Geometry: final body of the model. Coordinates: model frame, mm. Face numbers are marked on the shaded views. Coordinates: 2 decimals unless noted, no trailing zeros. Write each loop counter-clockwise with the first axis right and the second up, starting at its lowest first coordinate (ties: lowest second). Pieces come first, ordered by that corner, then holes. Notation, with made-up numbers: (57.25, -17) - (96.25, -17) arc R22 ccw to (96.25, 17) - close; hole circle Ø10 at (-7, 30.25). An arc over 180 degrees is marked (long way). Answer as a JSON object with one key per item and string values. Group by question number.
Item 1: First-contact query: pin 1 Ø4 at (x, y) = (-17, -8.5) entering from -Z; pin 2 Ø0.9 at (y, z) = (5.5, 3) entering from -X; pin 3 Ø1.5 at (x, z) = (-47, 3) entering from -Y; pin 4 Ø0.9 at (y, z) = (-6, 3.5) entering from +X. Flat tips, straight axial feed; report the tip coordinate or a pass-through.
Item 2: Section D-D on y = 37. Return loops of the section in (x, z), and give its area (3 significant figures).
Item 3: Section A-A on x = 0. Return loops of the section in (y, z).
Item 4: Line query: line 1 along X through (y, z) = (-54.5, 3.25); line 2 along X through (y, z) = (-43, 0.65); line 3 along Y through (x, z) = (40, 0.7). Output: solid intervals per line, ascending. Write a range as from..to.
Item 5: Section C-C on y = -42. Return loops of the section in (x, z).
Item 6: Section B-B on z = 4.05. State how many separate pieces and enclosed holes the cut face has, and give its area (3 significant figures).
Item 7: Mould query, pull axis Z, two halves, no side actions, for the marked faces 1 and 2. Classes: pulls with the +Z half, pulls with the -Z half, needs draft (parallel to the pull), parting line crosses it, or undercut.
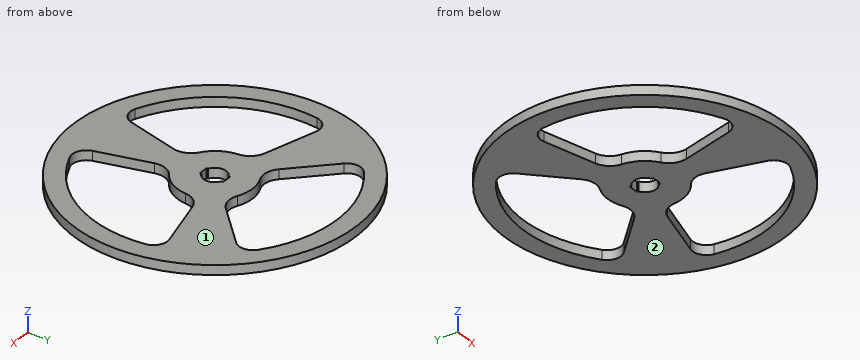
```python
from build123d import *

# Parameters (mm, degrees)
SKETCH1_R          = 75
SKETCH1_R_2        = 6
EXTRUSION1_DEPTH   = 5.1
CUT_EXTRUDE1_DEPTH = 107.188558706


with BuildPart() as part:
    # Sketch1 → Extrusion1 (new body)
    with BuildSketch(Plane.XY):
        Circle(SKETCH1_R)
        Circle(SKETCH1_R_2, mode=Mode.SUBTRACT)
        with BuildLine():
            ThreePointArc((40.502817464, 40.06150101), (42.745132776, 45.851099569), (39.856206804, 51.346691998))
            ThreePointArc((39.856206804, 51.346691998), (0, 65), (-39.856206804, 51.346691998))
            ThreePointArc((-39.856206804, 51.346691998), (-42.506769406, 45.932667816), (-40.316594862, 40.316594862))
            Line((-40.316594862, 40.316594862), (-20, 20))
            ThreePointArc((-20, 20), (-14.619951975, 17.215082215), (-8.619288125, 18.047378541))
            ThreePointArc((-8.619288125, 18.047378541), (0, 20), (8.619288125, 18.047378541))
            ThreePointArc((8.619288125, 18.047378541), (14.566416982, 17.206046598), (19.922803859, 19.923637571))
            Line((19.922803859, 19.923637571), (40.502817464, 40.06150101))
        make_face(mode=Mode.SUBTRACT)
        with BuildLine():
            ThreePointArc((-54.945686321, 15.045718344), (-61.080783406, 14.092821088), (-64.395643073, 8.843141592))
            ThreePointArc((-64.395643073, 8.843141592), (-56.291651246, -32.5), (-24.539436269, -60.18983359))
            ThreePointArc((-24.539436269, -60.18983359), (-18.525472489, -59.778276047), (-14.756897914, -55.073492776))
            Line((-14.756897914, -55.073492776), (-7.320508076, -27.320508076))
            ThreePointArc((-7.320508076, -27.320508076), (-7.598722539, -21.26879092), (-11.319844226, -16.48821175))
            ThreePointArc((-11.319844226, -16.48821175), (-17.320508076, -10), (-19.939132351, -1.559166791))
            ThreePointArc((-19.939132351, -1.559166791), (-22.184081943, 4.011863849), (-27.215778201, 7.291835471))
            Line((-27.215778201, 7.291835471), (-54.945686321, 15.045718344))
        make_face(mode=Mode.SUBTRACT)
        with BuildLine():
            ThreePointArc((14.442868856, -55.107219354), (18.33565063, -59.943920657), (24.539436269, -60.18983359))
            ThreePointArc((24.539436269, -60.18983359), (56.291651246, -32.5), (64.395643073, 8.843141592))
            ThreePointArc((64.395643073, 8.843141592), (61.032241895, 13.845608231), (55.073492776, 14.756897914))
            Line((55.073492776, 14.756897914), (27.320508076, 7.320508076))
            ThreePointArc((27.320508076, 7.320508076), (22.218674514, 4.053708705), (19.939132351, -1.559166791))
            ThreePointArc((19.939132351, -1.559166791), (17.320508076, -10), (11.319844226, -16.48821175))
            ThreePointArc((11.319844226, -16.48821175), (7.617664962, -21.217910447), (7.292974343, -27.215473042))
            Line((7.292974343, -27.215473042), (14.442868856, -55.107219354))
        make_face(mode=Mode.SUBTRACT)
    extrude(amount=EXTRUSION1_DEPTH)

    # Sketch2 → Cut-Extrude1 (cut, through all)
    with BuildSketch(Plane.XY.offset(5.1)):
        with BuildLine():
            ThreePointArc((-2.55, -5.431160097), (0, -6), (2.55, -5.431160097))
            Line((2.55, -5.431160097), (2.55, 5.431160097))
            ThreePointArc((2.55, 5.431160097), (0, 6), (-2.55, 5.431160097))
            Line((-2.55, 5.431160097), (-2.55, -5.431160097))
        make_face()
        with BuildLine():
            ThreePointArc((-2.55, 5.431160097), (0, 6), (2.55, 5.431160097))
            Line((2.55, 5.431160097), (2.55, 6.25))
            Line((2.55, 6.25), (-2.55, 6.25))
            Line((-2.55, 6.25), (-2.55, 5.431160097))
        make_face()
        with BuildLine():
            Line((-2.55, -6.25), (2.55, -6.25))
            Line((2.55, -6.25), (2.55, -5.431160097))
            ThreePointArc((2.55, -5.431160097), (0, -6), (-2.55, -5.431160097))
            Line((-2.55, -5.431160097), (-2.55, -6.25))
        make_face()
    extrude(amount=-CUT_EXTRUDE1_DEPTH, mode=Mode.SUBTRACT)


solid = part.part
```
Checks:
{
 "1": {"pin 1": "z = 0", "pin 2": "x = -74.83", "pin 3": "y = -59.04", "pin 4": "x = 74.79"},
 "2": {"outline": "(-65.24, 0) - (-37, 0) - (-37, 5.1) - (-65.24, 5.1) - close; (37.37, 0) - (65.24, 0) - (65.24, 5.1) - (37.37, 5.1) - close", "area": "286 mm^2"},
 "3": {"outline": "(-75, 0) - (-6.25, 0) - (-6.25, 5.1) - (-75, 5.1) - close; (6.25, 0) - (20, 0) - (20, 5.1) - (6.25, 5.1) - close; (65, 0) - (75, 0) - (75, 5.1) - (65, 5.1) - close"},
 "4": {"line 1": "-51.52..-35.42, -14.6..14.29, 35.42..51.52", "line 2": "-61.45..-48.74, -11.52..11.34, 48.74..61.45", "line 3": "-63.44..-51.23, 10.72..39.57, 51.23..63.44"},
 "5": {"outline": "(-62.14, 0) - (-49.61, 0) - (-49.61, 5.1) - (-62.14, 5.1) - close; (-11.25, 0) - (11.08, 0) - (11.08, 5.1) - (-11.25, 5.1) - close; (49.61, 0) - (62.14, 0) - (62.14, 5.1) - (49.61, 5.1) - close"},
 "6": {"separate pieces": "1", "enclosed holes": "4", "area": "8,680 mm^2"},
 "7": {"face 1": "pulls with the +Z half", "face 2": "pulls with the -Z half"}
}
